from build123d import *

# Parameters (mm, degrees)
SKETCH1_W             = 46
SKETCH1_H             = 40
BOSS_EXTRUDE1_DEPTH   = 4
SKETCH2_W             = 40
SKETCH2_H             = 45
BOSS_EXTRUDE2_DEPTH   = 5
BOSS_EXTRUDE3_DEPTH   = 20
SKETCH6_R             = 2.9
SKETCH6_R_2           = 1.55
SKETCH6_R_3           = 1.4
CUT_EXTRUDE2_DEPTH    = 9
FILLET1_R             = 2
FILLET2_R             = 2
CUT_EXTRUDE4_START    = -10
CUT_EXTRUDE4_DEPTH    = 10
SKETCH12_W            = 5
SKETCH12_H            = 40
CUT_EXTRUDE5_DEPTH    = 45
IZIM1_R               = 1.6
KES_EKSTR_ZYON1_DEPTH = 25
IZIM2_R               = 2.6
KES_EKSTR_ZYON2_DEPTH = 10
CUT_EXTRUDE11_DEPTH   = 15
SKETCH19_W            = 15
SKETCH19_H            = 40
CUT_EXTRUDE12_DEPTH   = 15
SKETCH20_R            = 1.4
SKETCH20_R_2          = 2.9
BOSS_EXTRUDE4_DEPTH   = 4


with BuildPart() as part:
    # Sketch1 → Boss-Extrude1 (new body)
    with BuildSketch(Plane(origin=(0, 0, 0), x_dir=(1, 0, 0), z_dir=(0, 1, 0))):
        Rectangle(SKETCH1_W, SKETCH1_H)
    extrude(amount=BOSS_EXTRUDE1_DEPTH)

    # Sketch2 → Boss-Extrude2 (add)
    with BuildSketch(Plane.ZY.offset(23)):
        with Locations((0, 26.5)):
            Rectangle(SKETCH2_W, SKETCH2_H)
    extrude(amount=-BOSS_EXTRUDE2_DEPTH)

    # Sketch3 → Boss-Extrude3 (add)
    with BuildSketch(Plane(origin=(23, 0, 0), x_dir=(0, 0, -1), z_dir=(1, 0, 0))):
        with BuildLine():
            Line((-20, 27), (-20, 2))
            Line((-20, 2), (20, 2))
            Line((20, 2), (20, 27))
            ThreePointArc((20, 27), (0, 47), (-20, 27))
        make_face()
    extrude(amount=-BOSS_EXTRUDE3_DEPTH)

    # Sketch6 → Cut-Extrude2 (cut)
    with BuildSketch(Plane(origin=(0, 4, 0), x_dir=(1, 0, 0), z_dir=(0, 1, 0))):
        with Locations(Location((0, 0, 0), (0, 0, 270))):
            Circle(SKETCH6_R)
        with Locations(Location((-4.99, 4.99, 0), (0, 0, 270))):
            Circle(SKETCH6_R_2)
        with Locations(Location((4.99, 4.99, 0), (0, 0, 270))):
            Circle(SKETCH6_R_3)
        with Locations(Location((-4.99, -4.98, 0), (0, 0, 270))):
            Circle(SKETCH6_R_2)
        with Locations(Location((4.99, -4.98, 0), (0, 0, 270))):
            Circle(SKETCH6_R_3)
    extrude(amount=-CUT_EXTRUDE2_DEPTH, mode=Mode.SUBTRACT)

    # Fillet1
    fillet1_edges = [part.edges().sort_by_distance(p)[0] for p in [
        (23, 0, 0),
    ]]
    fillet(fillet1_edges, radius=FILLET1_R)

    # Fillet2
    fillet2_edges = [part.edges().sort_by_distance(p)[0] for p in [
        (-23, 0, 0),
    ]]
    fillet(fillet2_edges, radius=FILLET2_R)

    # Sketch11 → Cut-Extrude4 (cut)
    with BuildSketch(Plane.ZY.offset(23).offset(CUT_EXTRUDE4_START)):
        with BuildLine():
            ThreePointArc((0, 47), (14.142135624, 41.142135624), (20, 27))
            Line((20, 27), (20, 47))
            Line((20, 47), (0, 47))
        make_face()
        with BuildLine():
            Line((-20, 47), (-20, 27))
            ThreePointArc((-20, 27), (-14.142135624, 41.142135624), (0, 47))
            Line((0, 47), (-20, 47))
        make_face()
    extrude(amount=CUT_EXTRUDE4_DEPTH, mode=Mode.SUBTRACT)


with BuildPart() as cut_extrude4_piece_1:
    # of the separate pieces the step leaves, piece 1, a body of its own (cut_extrude4_pieces)
    add(part.part.solids().sort_by_distance((-21, 0, -20))[0])

    # Çizim1 → Kes-Ekstrüzyon1 (cut)
    with BuildSketch(Plane(origin=(23, 0, 0), x_dir=(0, 0, -1), z_dir=(1, 0, 0))):
        with Locations((8, 27)):
            Circle(IZIM1_R)
        with Locations((0, 35)):
            Circle(IZIM1_R)
        with Locations((-8, 27)):
            Circle(IZIM1_R)
        with Locations((0, 19)):
            Circle(IZIM1_R)
    extrude(amount=-KES_EKSTR_ZYON1_DEPTH, mode=Mode.SUBTRACT)

    # Çizim2 → Kes-Ekstrüzyon2 (cut)
    with BuildSketch(Plane.ZY.offset(23)):
        with Locations((0, 27)):
            Circle(IZIM2_R)
    extrude(amount=-KES_EKSTR_ZYON2_DEPTH, mode=Mode.SUBTRACT)

    # Sketch18 → Cut-Extrude11 (cut)
    with BuildSketch(Plane(origin=(23, 0, 0), x_dir=(0, 0, -1), z_dir=(1, 0, 0))):
        with BuildLine():
            Line((-20, 27), (-20, 2))
            Line((-20, 2), (20, 2))
            Line((20, 2), (20, 27))
            ThreePointArc((20, 27), (0, 47), (-20, 27))
        make_face()
    extrude(amount=-CUT_EXTRUDE11_DEPTH, mode=Mode.SUBTRACT)

    # Sketch19 → Cut-Extrude12 (cut)
    with BuildSketch(Plane(origin=(0, 2, 0), x_dir=(1, 0, 0), z_dir=(0, 1, 0))):
        with Locations((15.5, 0)):
            Rectangle(SKETCH19_W, SKETCH19_H)
    extrude(amount=-CUT_EXTRUDE12_DEPTH, mode=Mode.SUBTRACT)

    # Sketch20 → Boss-Extrude4 (add)
    with BuildSketch(Plane(origin=(0, 0, 0), x_dir=(-1, 0, 0), z_dir=(0, -1, 0))):
        with Locations((-4.99, -4.98)):
            Circle(SKETCH20_R)
        with Locations((-4.99, 4.99)):
            Circle(SKETCH20_R)
        Circle(SKETCH20_R_2)
    extrude(amount=-BOSS_EXTRUDE4_DEPTH)


with BuildPart() as cut_extrude4_piece_2:
    # of the separate pieces the step leaves, piece 2, a body of its own (cut_extrude4_pieces)
    add(part.part.solids().sort_by_distance((-18, 47, -20))[0])

    # Sketch12 → Cut-Extrude5 (cut)
    with BuildSketch(Plane(origin=(0, 49, 0), x_dir=(1, 0, 0), z_dir=(0, 1, 0))):
        with Locations((-20.5, 0)):
            Rectangle(SKETCH12_W, SKETCH12_H)
    extrude(amount=-CUT_EXTRUDE5_DEPTH, mode=Mode.SUBTRACT)


solid = cut_extrude4_piece_1.part
CAD build for the part. Positions are in the model's coordinates, mm. A direction names the side the tool comes from. Give positions to 0.01 mm unless a question says otherwise; leave off trailing zeros. Loops run counter-clockwise (first coordinate to the right, second up) from the corner with the lowest first, then second, coordinate; pieces in that order, holes last. Notation, with made-up numbers: M -22,-7 L 5,-7 A28 cw 5,14 Z; hole C 60,66.25 d7. An arc over 180 degrees is marked long. One line per question, with ' | ' between items. Start each with the question number.
1. Two-plate mould, pull along X, no slides. Class faces 4 (the face through (-23, 20, 0)), 5 (the face through (-4.524, 2.028, 6.458)), 6 (the face through (8, 24, 0)), 7 (the face through (-6, 0, 0)): pulls with the +X half, pulls with the -X half, needs draft (parallel to the pull), parting line crosses it, or undercut.
2. Saw through at A-A on y = 19. Give the cut face in (x, z), plus the area to 3 significant figures.
3. Saw through at C-C on y = 43. Give the cut face in (x, z).
4. Flat gauge pin, fed straight in: pin 1 (6 mm diameter, centred on x = -4, z = -1, fed in from -Y). Where does the tip first touch, or does it go through?
5. Saw through at D-D on z = 4.98. Give the cut face in (x, y).
6. Saw through at B-B on x = -4.99. Give the cut face in (y, z).
7. Probe L1, parallel to Y at x = 6, z = 0; L2, parallel to X at y = 37.5, z = 16; L3, parallel to Y at x = -19.7, z = 0. List the from-to ranges inside material, lowest first. Write a range as from..to.
8. 3-axis set-ups, long thin cutter, end or side, ignore diameter. For faces 1 (the face through (-8, 4, 0)), 2 (the face through (5.535, 20.586, 0.208)), 3 (the face through (-20.535, 29.578, -0.338)): which of +Z, -Z, +X, -X, +Y, -Y reach the whole face in a straight line?
Result sheet:
1) face 4: pulls with the -X half | face 5: undercut | face 6: pulls with the +X half | face 7: needs draft
2) outline: M -23,-20 L -18,-20 L -18,20 L -23,20 Z; M 3,-20 L 8,-20 L 8,-1.6 L 3,-1.6 Z; M 3,1.6 L 8,1.6 L 8,20 L 3,20 Z | area: 384 mm^2
3) outline: M -23,-12 L -18,-12 L -18,12 L -23,12 Z; M 3,-12 L 8,-12 L 8,12 L 3,12 Z
4) pin 1: stops at y = 0
5) outline: M -23,2 A2 ccw -21,0 L -6.54,0 L -6.54,4 L -18,4 L -18,46.37 L -23,46.37 Z; M -3.44,0 L 8,0 L 8,46.37 L 3,46.37 L 3,4 L -3.44,4 Z
6) outline: M 0,-20 L 4,-20 L 4,-6.54 L 0,-6.54 Z; M 0,-3.44 L 4,-3.44 L 4,3.43 L 0,3.43 Z; M 0,6.53 L 4,6.53 L 4,20 L 0,20 Z
7) L1: y = 0..17.4, 20.6..33.4, 36.6..47 | L2: x = -23..-18, 3..8 | L3: y = 0..24.4, 29.6..47
8) face 1: +Z, -Z, +Y | face 2: +X | face 3: -X
